```python
from build123d import *

# Parameters (mm, degrees)
EXTRUDE_1_DEPTH     = 50
SKETCH_2_R          = 3
CUT_EXTRUDE_1_DEPTH = 4
SKETCH_3_R          = 8.9
SKETCH_3_R_2        = 2
CUT_EXTRUDE_2_DEPTH = 4


with BuildPart() as part:
    # Эскиз1 → Бобышка-Вытянуть1 (new body)
    with BuildSketch(Plane(origin=(0, 0, 0), x_dir=(1, 0, 0), z_dir=(0, 1, 0))):
        Polygon((0, 0), (50, 0), (50, 4), (4, 4), (4, 20.7), (0, 20.7), (0, 4), align=None)
    extrude(amount=EXTRUDE_1_DEPTH)

    # Эскиз2 → Вырез-Вытянуть1 (cut)
    with BuildSketch(Plane.ZY):
        with Locations((-10, 35)):
            Circle(SKETCH_2_R)
        with Locations((-10, 15)):
            Circle(SKETCH_2_R)
    extrude(amount=-CUT_EXTRUDE_1_DEPTH, mode=Mode.SUBTRACT)

    # Эскиз3 → Вырез-Вытянуть2 (cut)
    with BuildSketch(Plane(origin=(0, 0, -4), x_dir=(-1, 0, 0), z_dir=(0, 0, -1))):
        with Locations((-28, 25)):
            Circle(SKETCH_3_R)
        with Locations((-28, 39.5)):
            Circle(SKETCH_3_R_2)
        with Locations((-28, 10.5)):
            Circle(SKETCH_3_R_2)
    extrude(amount=-CUT_EXTRUDE_2_DEPTH, mode=Mode.SUBTRACT)


solid = part.part
```
Geometry check sheet. Reference: the model listing, model coordinates, mm. A direction names the side the tool comes from. Round coordinates to 2 decimals unless told otherwise and drop trailing zeros. Loops run counter-clockwise (first coordinate to the right, second up) from the corner with the lowest first, then second, coordinate; pieces in that order, holes last. Notation, with made-up numbers: (-26.75, 26.5) -> (18.25, 26.5) arc R9 ccw to (18.25, 36.5) -> close; hole circle Ø1 at (82.5, -15.75). An arc over 180 degrees is marked (long way). Use a Markdown table: item, result.
(1) Go/stop test with flat-tipped pins: P1, Ø6.5, axis at x = 28, y = 10.5, coming from the -Z side; P2, Ø5, axis at y = 31, z = -13, coming from the +X side. Record where each tip stops, or that it passes through.
Calculated:
| item | result |
|---|---|
| P1 | z = -4 |
| P2 | x = 4 |
(2) Sectioned sample at A-A (z = -10). Enter the section's corners in (x, y), then the cut area to 3 significant figures.
Calculated:
| item | result |
|---|---|
| outline | (0, 0) -> (4, 0) -> (4, 12) -> (0, 12) -> close; (0, 18) -> (4, 18) -> (4, 32) -> (0, 32) -> close; (0, 38) -> (4, 38) -> (4, 50) -> (0, 50) -> close |
| area | 152 mm² |
(3) Sectioned sample at B-B (y = 39.5). Enter the section's corners in (x, z), then the cut area to 3 significant figures.
Calculated:
| item | result |
|---|---|
| outline | (0, -20.7) -> (4, -20.7) -> (4, -4) -> (26, -4) -> (26, 0) -> (0, 0) -> close; (30, -4) -> (50, -4) -> (50, 0) -> (30, 0) -> close |
| area | 251 mm² |
(4) Sectioned sample at C-C (x = 22). Enter the section's corners in (y, z), then the cut area to 3 significant figures.
Calculated:
| item | result |
|---|---|
| outline | (0, -4) -> (18.43, -4) -> (18.43, 0) -> (0, 0) -> close; (31.57, -4) -> (50, -4) -> (50, 0) -> (31.57, 0) -> close |
| area | 147 mm² |
(5) Mould release check, pull along X, two halves, no side actions. Record for faces 3 (the flat face through (0, 25, -10)), 4 (the flat face through (50, 25, -2)), 5 (the cylindrical face through (35.06, 19.58, -2.03)), 6 (the cylindrical face through (1.97, 37.03, -12.21)): released by +X, released by -X, zero draft, split by the parting line, or undercut.
Calculated:
| item | result |
|---|---|
| face 3 | released by -X |
| face 4 | released by +X |
| face 5 | undercut |
| face 6 | zero draft |
(6) Set-up check for faces 1 (the flat face through (19, 19, 0)), 2 (the flat face through (4, 25, -12)): record each of +Z, -Z, +X, -X, +Y, -Y from which the full face is reachable in a straight line by a thin tool's end or side.
Calculated:
| item | result |
|---|---|
| face 1 | +Z, +X, -X, +Y, -Y |
| face 2 | -Z, +X, +Y, -Y |
(7) Scan lines: probe 1 along Y at (x, z) = (28, -1.1); probe 2 along Y at (x, z) = (2.6, -10); probe 3 along X at (y, z) = (4, -13.75). Record each from-to range of solid material in increasing order.
Calculated:
| item | result |
|---|---|
| probe 1 | 0 to 8.5, 12.5 to 16.1, 33.9 to 37.5, 41.5 to 50 |
| probe 2 | 0 to 12, 18 to 32, 38 to 50 |
| probe 3 | 0 to 4 |
(8) Sectioned sample at D-D (y = 15). Enter the section's corners in (x, z), then the cut area to 3 significant figures.
Calculated:
| item | result |
|---|---|
| outline | (0, -20.7) -> (4, -20.7) -> (4, -13) -> (0, -13) -> close; (0, -7) -> (4, -7) -> (4, -4) -> (50, -4) -> (50, 0) -> (0, 0) -> close |
| area | 243 mm² |
